Work out the finished part from the listing and answer in its coordinate system (mm). Face numbers are marked on the shaded views. A direction names the side the tool comes from. Coordinates: 2 decimals unless noted, no trailing zeros. Loops run counter-clockwise (first coordinate to the right, second up) from the corner with the lowest first, then second, coordinate; pieces in that order, holes last. Notation, with made-up numbers: (80, 26) -> (85, 26) arc R11 cw to (85, 47) -> close; hole circle Ø10 at (-36.5, 35). An arc over 180 degrees is marked (long way). Use a Markdown table: item, result.
from build123d import *

# Parameters (mm, degrees)
EXTRUDE_1_DEPTH     = 5
EXTRUDE_2_DEPTH     = 20
CUT_EXTRUDE_1_DEPTH = 45


with BuildPart() as part:
    # Sketch 1 → Extrude 1 (new body)
    with BuildSketch(Plane(origin=(0, 0, 0), x_dir=(1, 0, 0), z_dir=(0, 1, 0))):
        Polygon((-10, -10), (-5, 10), (-15, 10), (-15, -10), align=None)
        Polygon((5, 10), (-5, 10), (-10, -10), (10, -10), align=None)
        Polygon((15, 10), (5, 10), (10, -10), (15, -10), align=None)
    extrude(amount=EXTRUDE_1_DEPTH)

    # Sketch 1_3 → Extrude 2 (add)
    with BuildSketch(Plane(origin=(0, 0, 0), x_dir=(1, 0, 0), z_dir=(0, 1, 0))):
        Polygon((-10, -10), (-5, 10), (-15, 10), (-15, -10), align=None)
        Polygon((15, 10), (5, 10), (10, -10), (15, -10), align=None)
    extrude(amount=EXTRUDE_2_DEPTH)

    # Sketch 2 → Cut-Extrude 1 (cut)
    with BuildSketch(Plane(origin=(15, 0, 0), x_dir=(0, 0, -1), z_dir=(1, 0, 0))):
        Polygon((10, 20), (-10, 5), (-10, 20), align=None)
    extrude(amount=-CUT_EXTRUDE_1_DEPTH, mode=Mode.SUBTRACT)


solid = part.part
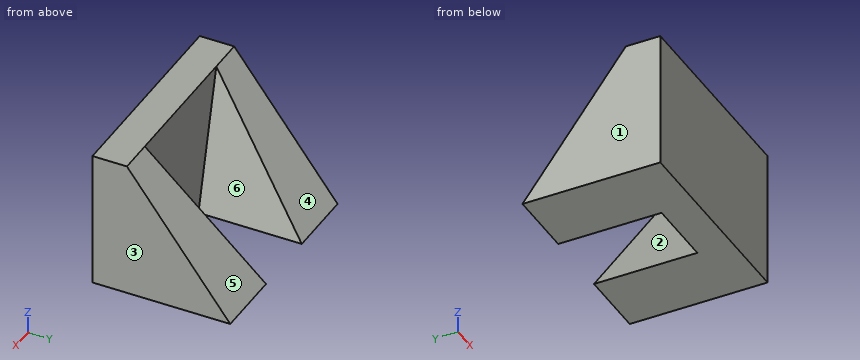
Q1. Consider line 1 (Y direction, x = 3.5, z = 0); line 2 (Z direction, x = 13.25, y = 8.75); line 3 (X direction, y = 15, z = -6). Determine where each line is inside the solid, lowest interval first. Write a range as [from, to].
Solved:
| item | result |
|---|---|
| line 1 | [0, 5] |
| line 2 | [-10, 5] |
| line 3 | [-15, -6], [6, 15] |
Q2. Determine the mould class of the marked faces 1, 2, 3 and 4 for opening direction X: pulls with the +X half, pulls with the -X half, needs draft (parallel to the pull), parting line crosses it, or undercut.
Solved:
| item | result |
|---|---|
| face 1 | pulls with the -X half |
| face 2 | undercut |
| face 3 | pulls with the +X half |
| face 4 | needs draft |
Q3. Section D-D on x = 6.75 is taken. Determine the outline of the cut face in (y, z).
Solved:
| item | result |
|---|---|
| outline | (0, -10) -> (20, -10) -> (14.75, -3) -> (5, -3) -> (5, 10) -> (0, 10) -> close |
Q4. Section B-B on z = -6 is taken. Determine the outline of the cut face in (x, y).
Solved:
| item | result |
|---|---|
| outline | (-15, 0) -> (15, 0) -> (15, 17) -> (6, 17) -> (6, 5) -> (-6, 5) -> (-6, 17) -> (-15, 17) -> close |
Q5. Section C-C on y = 7.25 is taken. Determine the outline of the cut face in (x, z).
Solved:
| item | result |
|---|---|
| outline | (-15, -10) -> (-5, -10) -> (-9.25, 7) -> (-15, 7) -> close; (5, -10) -> (15, -10) -> (15, 7) -> (9.25, 7) -> close |
Q6. For the marked faces 5 and 6, determine the directions among +Z, -Z, +X, -X, +Y, -Y from which every point of the face is accessible in a straight line to the end or side of a thin tool.
Solved:
| item | result |
|---|---|
| face 5 | +Z, +X, -X, +Y |
| face 6 | +Z, +Y |
Q7. Section A-A on y = 14.75 is taken. Determine the outline of the cut face in (x, z).
Solved:
| item | result |
|---|---|
| outline | (-15, -10) -> (-5, -10) -> (-6.75, -3) -> (-15, -3) -> close; (5, -10) -> (15, -10) -> (15, -3) -> (6.75, -3) -> close |
